Autodesk Inventor part; units mm, degrees
ref_plane "Plano inicial" through (0, 0, 0) normal (0, 0, 1) x (1, 0, 0)
ref_plane "Plano final" through (0, 0, 550) normal (0, 0, 1) x (1, 0, 0)
ref_plane "Plano de trabalho4" through (-15, 0, 550) normal (0.7071, 0, 0.7071) x (0.7071, 0, -0.7071)
ref_plane "Plano inicial" through (0, 0, 0) normal (0, 0, 1) x (1, 0, 0)
ref_plane "Plano final" through (0, 0, 550) normal (0, 0, 1) x (1, 0, 0)
sketch "Esboço" plane through (0, 0, 0) normal (0, 0, 1) x (1, 0, 0)
  line L0 (-15, -11) -> (-15, 11)
  line L1 (-11, 15) -> (11, 15)
  line L2 (15, 11) -> (15, -11)
  line L3 (11, -15) -> (-11, -15)
  arc A0 (-15, -11) -> (-11, -15) centre (-11, -11) ccw
  arc A1 (15, 11) -> (11, 15) centre (11, 11) ccw
  arc A2 (-11, 15) -> (-15, 11) centre (-11, 11) ccw
  arc A3 (11, -15) -> (15, -11) centre (11, -11) ccw
  arc A4 (-11, 13) -> (-13, 11) centre (-11, 11) ccw
  line L4 (-11, 13) -> (11, 13)
  arc A5 (13, 11) -> (11, 13) centre (11, 11) ccw
  line L5 (13, 11) -> (13, -11)
  arc A6 (11, -13) -> (13, -11) centre (11, -11) ccw
  line L6 (11, -13) -> (-11, -13)
  arc A7 (-13, -11) -> (-11, -13) centre (-11, -11) ccw
  line L7 (-13, -11) -> (-13, 11)
  line L8 (0, 22.1598) -> (0, -22.1598) construction
  line L9 (-22.1598, 0) -> (22.1598, 0) construction
  dimension "d7" = 4
  dimension "d9" = 30
  dimension "d11" = 30
  dimension "d12" = 2
  dimension "d15" = 15
  dimension "d16" = 15
extrude "Corpo" add sketch "Esboço" along normal up to surface (550 mm away) from surface at 0
sketch "Sketch3" plane through (0, 0, 0) normal (0, 0, 1) x (1, 0, 0)
  line L0 (0, 0) -> (10, 0)
ref_plane "Work Plane3" through (0, 0, 0) normal (0, -1, 0) x (1, 0, 0)
sketch "Sketch4" plane through (0, 0, 0) normal (0, -1, 0) x (1, 0, 0)
  line L0 (-2, 0) -> (12, 0)
  line L1 (-2, 550) -> (12, 550)
  dimension "d18" = 550
ref_plane "Plano de trabalho4" through (-15, 0, 550) normal (0.7071, 0, 0.7071) x (0.7071, 0, -0.7071)
split "Dividir1" plane through (-15, 0, 550) removes the side toward (0.7071, 0, 0.7071)
equation "\"d7\" = G_IR"
equation "\"d9\" = G_W"
equation "\"d11\" = G_H"
equation "\"d12\" = G_T"
equation "\"d15\" = 0.5 * d9"
equation "\"d16\" = 0.5 * d11"
equation "\"d3\" = G_L"
equation "\"G_W\" = 30"
equation "\"G_H\" = 30"
equation "\"G_T\" = 2"
equation "\"G_IR\" = 4"
equation "\"G_L\" = d18"
equation "\"G_OFFSET_START\" = 0"
equation "\"G_OFFSET_END\" = 0"
properties part number "ISO 10799-2 - 30x30x2 - 550" material "Aço, suave"
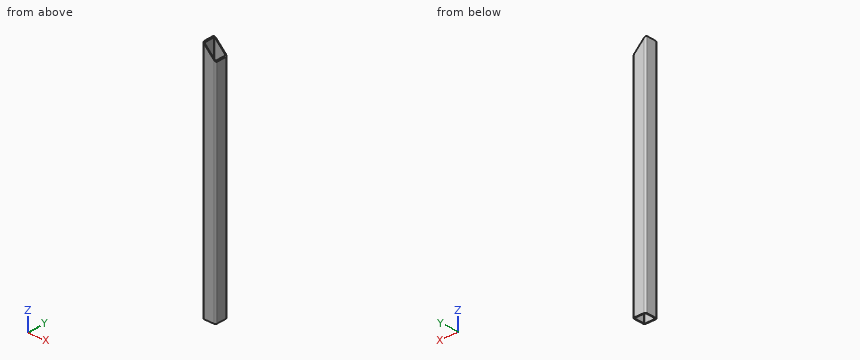
Design review of the part built by this model. Coordinates are the model's own, in mm. Round coordinates to 2 decimals unless told otherwise and drop trailing zeros. Write each loop counter-clockwise with the first axis right and the second up, starting at its lowest first coordinate (ties: lowest second). Pieces come first, ordered by that corner, then holes.
Item 1: Consider section C-C on z = 156.5. Give the boundary of the cut face in (x, y).
Item 2: Consider section B-B on y = 2. Give the boundary of the cut face in (x, z).
Item 3: For pin 1 Ø10 at (x, y) = (-5, -4.5) entering from +Z, flat-tipped, find the tip position at first contact; note if it passes through.
Item 4: Wall thickness on L1, parallel to X at y = -2.5, z = 71; L2, parallel to X at y = -12.25, z = 82.5: over which ranges is each line inside the solid? List them lowest first.
Item 5: Consider section A-A on x = 5.5. Give the boundary of the cut face in (y, z), and give its area (3 significant figures).
Check values:
1. outline: (-15, -11) arc R4 ccw to (-11, -15) - (11, -15) arc R4 ccw to (15, -11) - (15, 11) arc R4 ccw to (11, 15) - (-11, 15) arc R4 ccw to (-15, 11) - close; hole (-13, -11) arc R2 ccw to (-11, -13) - (11, -13) arc R2 ccw to (13, -11) - (13, 11) arc R2 ccw to (11, 13) - (-11, 13) arc R2 ccw to (-13, 11) - close
2. outline: (-15, 0) - (-13, 0) - (-13, 548) - (-15, 550) - close; (13, 0) - (15, 0) - (15, 520) - (13, 522) - close
3. pin 1: passes through
4. L1: x = -15 to -13, 13 to 15
4. L2: x = -14.8 to -12.56, 12.56 to 14.8
5. outline: (-15, 0) - (-13, 0) - (-13, 529.5) - (-15, 529.5) - close; (13, 0) - (15, 0) - (15, 529.5) - (13, 529.5) - close
5. area: 2,120 mm2
